```python
from build123d import *

# Parameters (mm, degrees)
F1_DEPTH = 4
F2_R     = 4.5
F3_DEPTH = 40
F4_DEPTH = 25


with BuildPart() as f1:
    # F0 (on Top) → F1 (new body)
    with BuildSketch(Plane.XY):
        with BuildLine():
            Line((-25, -30), (25, -30))
            ThreePointArc((25, -30), (28.535534, -28.535534), (30, -25))
            Line((30, -25), (30, 25))
            ThreePointArc((30, 25), (28.535534, 28.535534), (25, 30))
            Line((25, 30), (-25, 30))
            ThreePointArc((-25, 30), (-28.535534, 28.535534), (-30, 25))
            Line((-30, 25), (-30, -25))
            ThreePointArc((-30, -25), (-28.535534, -28.535534), (-25, -30))
        make_face()
    extrude(amount=F1_DEPTH)

    # F2 (on face) → F3 (join)
    with BuildSketch(Plane.XY.offset(4)):
        with BuildLine():
            Line((-30, 25), (-7.574446, 2.574446))
            ThreePointArc((-7.574446, 2.574446), (-8, 0), (-7.574446, -2.574446))
            Line((-7.574446, -2.574446), (-30, -25))
            ThreePointArc((-30, -25), (-28.535534, -28.535534), (-25, -30))
            Line((-25, -30), (-2.574446, -7.574446))
            ThreePointArc((-2.574446, -7.574446), (0, -8), (2.574446, -7.574446))
            Line((2.574446, -7.574446), (25, -30))
            ThreePointArc((25, -30), (28.535534, -28.535534), (30, -25))
            Line((30, -25), (7.574446, -2.574446))
            ThreePointArc((7.574446, -2.574446), (8, 0), (7.574446, 2.574446))
            Line((7.574446, 2.574446), (30, 25))
            ThreePointArc((30, 25), (28.535534, 28.535534), (25, 30))
            Line((25, 30), (2.574446, 7.574446))
            ThreePointArc((2.574446, 7.574446), (0, 8), (-2.574446, 7.574446))
            Line((-2.574446, 7.574446), (-25, 30))
            ThreePointArc((-25, 30), (-28.535534, 28.535534), (-30, 25))
        make_face()
        Circle(F2_R, mode=Mode.SUBTRACT)
    extrude(amount=F3_DEPTH)

    # F2 (on face) → F4 (cut)
    with BuildSketch(Plane.XY.offset(4)):
        Circle(F2_R)
    extrude(amount=-F4_DEPTH, mode=Mode.SUBTRACT)


solid = f1.part
```
Check sheet for the modelled part. Datum: model origin and axes. Units: mm. A direction names the side the tool comes from. Give positions to 0.01 mm unless a question says otherwise; leave off trailing zeros. Write each loop counter-clockwise with the first axis right and the second up, starting at its lowest first coordinate (ties: lowest second). Pieces come first, ordered by that corner, then holes.
Item 1: Access from +Z, -Z, +X, -X, +Y, -Y to the whole of each face (thin tool, end or side, straight path). Record for faces 1 (the face through (19, 14, 24)), 2 (the face through (0, -21, 4)), 3 (the face through (-19, -14, 24)).
Item 2: Draft check along X on faces 4 (the face through (19, -14, 24)), 5 (the face through (-14, -19, 24)), 6 (the face through (0, 7, 0)), 7 (the face through (-28, 29, 22)). Enter one of: released by +X, released by -X, zero draft, split by the parting line, or undercut.
Item 3: Scan lines: L1, parallel to Y at x = 0, z = 1.9; L2, parallel to Z at x = 23, y = -3; L3, parallel to Y at x = -10, z = 12. Record each from-to range of solid material in increasing order.
Item 4: Cross-section at A-A (x = 0). Enter the section's corners in (y, z), and give its area (3 significant figures).
Item 5: Cross-section at D-D (x = -19.5). Enter the section's corners in (y, z), and give its area (3 significant figures).
Item 6: Cross-section at C-C (z = 3). Enter the section's corners in (x, y).
Item 7: Gauge pin test, flat ends, axial feed: pin 1 (1 mm diameter, centred on x = -10, y = 21, fed in from +Z); pin 2 (6 mm diameter, centred on y = -5.5, z = 12, fed in from -X); pin 3 (5 mm diameter, centred on x = 3, z = 32, fed in from +Y). Record the tip position at first contact, or that the pin passes through.
Report:
1. face 1: +Z, +X
1. face 2: +Z, -Y
1. face 3: +Z, -X
2. face 4: released by +X
2. face 5: undercut
2. face 6: zero draft
2. face 7: released by -X
3. L1: y = -30 to -4.5, 4.5 to 30
3. L2: z = 0 to 4
3. L3: y = -15 to -5, 5 to 15
4. outline: (-30, 0) - (-4.5, 0) - (-4.5, 44) - (-8, 44) - (-8, 4) - (-30, 4) - close; (4.5, 0) - (30, 0) - (30, 4) - (8, 4) - (8, 44) - (4.5, 44) - close
4. area: 484 mm2
5. outline: (-30, 0) - (30, 0) - (30, 4) - (24.5, 4) - (24.5, 44) - (14.5, 44) - (14.5, 4) - (-14.5, 4) - (-14.5, 44) - (-24.5, 44) - (-24.5, 4) - (-30, 4) - close
5. area: 1,040 mm2
6. outline: (-30, -25) arc R5 ccw to (-25, -30) - (25, -30) arc R5 ccw to (30, -25) - (30, 25) arc R5 ccw to (25, 30) - (-25, 30) arc R5 ccw to (-30, 25) - close; hole circle Ø9 at (0, 0)
7. pin 1: stops at z = 4
7. pin 2: stops at x = -13.5
7. pin 3: stops at y = 10.5
